Geometry: final body of the model. Coordinates: model frame, mm. A direction names the side the tool comes from. Coordinates: 2 decimals unless noted, no trailing zeros. Order: outer loops, then holes, each group sorted by start corner. A loop starts at its lowest first (then second) coordinate and runs counter-clockwise, first axis right, second up. Notation, with made-up numbers: M 34.5,16.25 L 40.5,16.25 A24 ccw 40.5,47.25 Z; hole C -39.75,48 d3. An arc over 180 degrees is marked long. One line per question, with ' | ' between items.
from build123d import *

# Parameters (mm, degrees)
F1_DEPTH = 10
F2_R     = 9
F3_DEPTH = 8
F4_R     = 3.4
F5_DEPTH = 25


with BuildPart() as f1:
    # F0 (on Top) → F1 (new body)
    with BuildSketch(Plane.XY):
        Polygon((6.928203, 12), (-6.928203, 12), (-13.856406, 0), (-6.928203, -12), (6.928203, -12), (13.856406, 0), align=None)
    extrude(amount=F1_DEPTH)

    # F2 (on face) → F3 (join)
    with BuildSketch(Plane(origin=(0, 0, 0), x_dir=(1, 0, 0), z_dir=(0, 0, -1))):
        Circle(F2_R)
    extrude(amount=F3_DEPTH)

    # F4 (on face) → F5 (cut)
    with BuildSketch(Plane.XY.offset(10)):
        Circle(F4_R)
    extrude(amount=-F5_DEPTH, mode=Mode.SUBTRACT)


solid = f1.part
1. Section B-B, the plane z = 5.75. Output: boundary loops of the cut face in (x, y).
Response values:
outline: M -13.86,0 L -6.93,-12 L 6.93,-12 L 13.86,0 L 6.93,12 L -6.93,12 Z; hole C 0,0 d6.8
2. Draft query along X for faces 3 (the face through (0, -12, 5)), 4 (the face through (10.44, 5.92, 4.93)), 5 (the face through (-0.74, -3.32, 1.13)). Return one class per face: pulls with the +X half, pulls with the -X half, needs draft (parallel to the pull), parting line crosses it, or undercut.
Response values:
face 3: needs draft | face 4: pulls with the +X half | face 5: undercut
3. Material intervals for line 1 (Y direction, x = 0, z = 0.75); line 2 (Y direction, x = 0, z = -1.25); line 3 (Z direction, x = -9.25, y = -7.5), sorted ascending. Write a range as [from, to].
Response values:
line 1: y = [-12, -3.4], [3.4, 12] | line 2: y = [-9, -3.4], [3.4, 9] | line 3: z = [0, 10]
4. Access query for faces 1 (the face through (-1.172, -8.923, -3.944)), 2 (the face through (0, 12, 5)). Directions: +Z, -Z, +X, -X, +Y, -Y. A direction counts if a zero-diameter tool reaches every point of the face in a straight line with its end or side. Return the directions, or none.
Response values:
face 1: -Z | face 2: +Z, -Z, +X, -X, +Y
5. Pin query (flat end, axial travel): P1, Ø1.5, axis at y = -9, z = -6, coming from the +X side. Return the tip coordinate at first contact, or that it passes through.
Response values:
P1: stops at x = 3.6
6. Section D-D, the plane y = -4.25. Output: boundary loops of the cut face in (x, z).
Response values:
outline: M -11.4,0 L -7.93,0 L -7.93,-8 L 7.93,-8 L 7.93,0 L 11.4,0 L 11.4,10 L -11.4,10 Z
7. Section A-A, the plane x = 0. Output: boundary loops of the cut face in (y, z), and give its area (3 significant figures).
Response values:
outline: M -12,0 L -9,0 L -9,-8 L -3.4,-8 L -3.4,10 L -12,10 Z; M 3.4,-8 L 9,-8 L 9,0 L 12,0 L 12,10 L 3.4,10 Z | area: 262 mm^2
8. Section C-C, the plane y = 2.25. Output: boundary loops of the cut face in (x, z).
Response values:
outline: M -12.56,0 L -8.71,0 L -8.71,-8 L -2.55,-8 L -2.55,10 L -12.56,10 Z; M 2.55,-8 L 8.71,-8 L 8.71,0 L 12.56,0 L 12.56,10 L 2.55,10 Z
